Read the model definition and answer for the solid it produces. Units are mm, in the model's axes. A direction names the side the tool comes from. Coordinates: 2 decimals unless noted, no trailing zeros. Order: outer loops, then holes, each group sorted by start corner. A loop starts at its lowest first (then second) coordinate and runs counter-clockwise, first axis right, second up. Notation, with made-up numbers: (46.25, 19) - (58.25, 19) arc R25 ccw to (58.25, 40) - close; hole circle Ø1 at (30.25, 52.5). An arc over 180 degrees is marked (long way). Write item = value, one per line.
from build123d import *

# Parameters (mm, degrees)
SKETCH1_R           = 4.1275
BOSS_EXTRUDE2_DEPTH = 4.064
SKETCH2_R           = 4.8895
BOSS_EXTRUDE3_DEPTH = 1.5875
SKETCH7_W           = 4.5
SKETCH7_H           = 3.5
CUT_EXTRUDE2_DEPTH  = 6.6515
CHAMFER1_SIZE       = 1
SKETCH8_R           = 4.8895
CUT_EXTRUDE3_DEPTH  = 0.9


with BuildPart() as part:
    # Sketch1 → Boss-Extrude2 (new body)
    with BuildSketch(Plane.XY):
        with Locations((6.731, -165.7192297)):
            Circle(SKETCH1_R)
    extrude(amount=-BOSS_EXTRUDE2_DEPTH)

    # Sketch2 → Boss-Extrude3 (add)
    with BuildSketch(Plane.XY):
        with Locations((6.731, -165.7192297)):
            Circle(SKETCH2_R)
    extrude(amount=BOSS_EXTRUDE3_DEPTH)

    # Sketch7 → Cut-Extrude2 (cut, through all)
    with BuildSketch(Plane(origin=(0, 0, -4.064), x_dir=(-1, 0, 0), z_dir=(0, 0, -1))):
        with Locations((-6.731, -165.7192297)):
            Rectangle(SKETCH7_W, SKETCH7_H)
    extrude(amount=-CUT_EXTRUDE2_DEPTH, mode=Mode.SUBTRACT)

    # Chamfer1
    chamfer1_edges = [part.edges().sort_by_distance(p)[0] for p in [
        (4.481, -163.9692297, -1.23825),
        (4.481, -167.4692297, -1.23825),
        (8.981, -167.4692297, -1.23825),
        (8.981, -163.9692297, -1.23825),
    ]]
    chamfer(chamfer1_edges, length=CHAMFER1_SIZE)

    # Sketch8 → Cut-Extrude3 (cut)
    with BuildSketch(Plane.XY.offset(1.5875)):
        with Locations((6.731, -165.7192297)):
            Circle(SKETCH8_R)
    extrude(amount=-CUT_EXTRUDE3_DEPTH, mode=Mode.SUBTRACT)


solid = part.part
1) The part is cut by section B-B (y = -167). Determine the outline of the cut face in (x, z), and give its area (3 significant figures).
Returned:
outline = (2.01, 0) - (2.81, 0) - (2.81, -4.06) - (5.01, -4.06) - (5.01, 0.69) - (2.01, 0.69) - close; (8.45, -4.06) - (10.65, -4.06) - (10.65, 0) - (11.45, 0) - (11.45, 0.69) - (8.45, 0.69) - close
area = 22.0 mm^2
2) The part is cut by section C-C (z = -2.4). Determine the outline of the cut face in (x, y) (1 decimal).
Returned:
outline = circle Ø8.3 at (6.7, -165.7); hole (4.5, -166.5) - (5.5, -167.5) - (8, -167.5) - (9, -166.5) - (9, -165) - (8, -164) - (5.5, -164) - (4.5, -165) - close
3) Determine the mould class of faces 1 (the face through (3, -168, 0)), 2 (the face through (3.13, -162.41, 0.34)), 3 (the face through (4.97, -164.48, -1.72)), 4 (the face through (4.99, -166.98, -1.72)) for opening direction X: pulls with the +X half, pulls with the -X half, needs draft (parallel to the pull), parting line crosses it, or undercut.
Returned:
face_1 = needs draft
face_2 = parting line crosses it
face_3 = undercut
face_4 = undercut
4) The part is cut by section A-A (x = 6.75). Determine the outline of the cut face in (y, z).
Returned:
outline = (-170.61, 0) - (-169.85, 0) - (-169.85, -4.06) - (-167.47, -4.06) - (-167.47, 0.69) - (-170.61, 0.69) - close; (-163.97, -4.06) - (-161.59, -4.06) - (-161.59, 0) - (-160.83, 0) - (-160.83, 0.69) - (-163.97, 0.69) - close
5) For faces 5 (the face through (4.481, -166, -2)), 6 (the face through (3.69, -162.93, -2)), 7 (the face through (7, -168, 0.687)), determine the directions among +Z, -Z, +X, -X, +Y, -Y from which every point of the face is accessible in a straight line to the end or side of a thin tool.
Returned:
face_5 = +Z, -Z
face_6 = -Z
face_7 = +Z, +X, -X, +Y, -Y
6) Flat-ended cylindrical pins translate along their axes: pin 1 Ø2 at (x, z) = (10.5, -2.5) entering from -Y; pin 2 Ø2 at (x, z) = (6, -2) entering from -Y; pin 3 Ø1.2 at (y, z) = (-165.5, -1.5) entering from -X. Find the tip coordinate at first contact, or state that the pin passes through.
Returned:
pin_1 = -168.78
pin_2 = -169.85
pin_3 = 2.6
7) Straight lines are drawn through the part: line 1 along Y through (x, z) = (8, -1); line 2 along Z through (x, y) = (11.25, -165.75); line 3 along X through (y, z) = (-166.5, -0.15). For each, find the intervals that lie inside material, in ascending order. Write a range as from..to.
Returned:
line_1 = -169.65..-167.45, -163.99..-161.79
line_2 = 0..0.69
line_3 = 2.68..4.51, 8.95..10.78
8) The part is cut by section D-D (y = -162.5). Determine the outline of the cut face in (x, z), and give its area (3 significant figures).
Returned:
outline = (3.05, 0) - (4.15, 0) - (4.15, -4.06) - (9.31, -4.06) - (9.31, 0) - (10.41, 0) - (10.41, 0.69) - (3.05, 0.69) - close
area = 26.1 mm^2
